Input: part model. Units: mm. Frame: model coordinates. Face numbers are marked on the shaded views. A direction names the side the tool comes from. Coordinates: 2 decimals unless noted, no trailing zeros. Order: outer loops, then holes, each group sorted by start corner. A loop starts at its lowest first (then second) coordinate and runs counter-clockwise, first axis right, second up. Notation, with made-up numbers: M 76,5.25 L 85,5.25 A5 cw 85,11.25 Z; hole C 44,55 d1. An arc over 180 degrees is marked long. Answer in a Markdown table with one row per item.
Autodesk Inventor part; units mm, degrees
ref_plane "YZ Plane" through (0, 0, 0) normal (1, 0, 0) x (0, 1, 0)
ref_plane "XZ Plane" through (0, 0, 0) normal (0, 1, 0) x (-1, 0, 0)
ref_plane "XY Plane" through (0, 0, 0) normal (0, 0, 1) x (1, 0, 0)
sketch "스케치1" plane through (0, 0, 0) normal (0, 0, 1) x (1, 0, 0)
  line L0 (-46, -31.5) -> (46, -31.5)
  line L1 (46, -31.5) -> (46, 31.5)
  line L2 (46, 31.5) -> (-46, 31.5)
  line L3 (-46, 31.5) -> (-46, -31.5)
  line L4 (-46, -31.5) -> (46, 31.5) construction
  line L5 (46, -31.5) -> (-46, 31.5) construction
  line L6 (-42.5, 28) -> (42.5, 28) construction
  line L7 (42.5, 28) -> (42.5, -28) construction
  line L8 (42.5, -28) -> (-42.5, -28) construction
  line L9 (-42.5, -28) -> (-42.5, 28) construction
  line L10 (-42.5, 28) -> (42.5, -28) construction
  line L11 (42.5, 28) -> (-42.5, -28) construction
  circle A0 centre (-39, -24.5) radius 1
  circle A1 centre (19, -24.5) radius 1
  line L12 (0, 0) -> (14.8173, 0)
  circle A2 centre (-39, 24.5) radius 1
  circle A3 centre (19, 24.5) radius 1
  line L13 (-46, 31.5) -> (-41, 31.5)
  line L14 (-41, 31.5) -> (-41, 34)
  line L15 (-41, 34) -> (-46, 34) construction
  line L16 (-46, 34) -> (-46, 31.5)
  circle A4 centre (-43.5, 34) radius 2.5
  circle A5 centre (-43.5, 34) radius 1.25
  line L17 (0, 0) -> (0, 10.4922)
  line L18 (46, 31.5) -> (41, 31.5)
  line L19 (41, 31.5) -> (41, 34)
  line L20 (41, 34) -> (46, 34) construction
  line L21 (46, 34) -> (46, 31.5)
  circle A6 centre (43.5, 34) radius 2.5
  circle A7 centre (43.5, 34) radius 1.25
  line L22 (46, -31.5) -> (-46, -31.5)
  line L23 (-46, -31.5) -> (-41, -31.5)
  line L24 (-41, -31.5) -> (-41, -34)
  line L25 (-41, -34) -> (-46, -34) construction
  line L26 (-46, -34) -> (-46, -31.5)
  circle A8 centre (-43.5, -34) radius 2.5
  circle A9 centre (-43.5, -34) radius 1.25
  line L27 (41, -31.5) -> (41, -34)
  circle A10 centre (43.5, -34) radius 1.25
  line L28 (41, -34) -> (46, -34) construction
  line L29 (46, -34) -> (46, -31.5)
  circle A11 centre (43.5, -34) radius 2.5
  line L30 (46, -31.5) -> (41, -31.5)
  dimension "d0" = 92
  dimension "d1" = 63
  dimension "d2" = 85
  dimension "d3" = 56
  dimension "d4" = 3.5
  dimension "d5" = 3.5
  dimension "d6" = 2
  dimension "d7" = 2
  dimension "d8" = 58
  dimension "d9" = 3.5
  dimension "d10" = 5
  dimension "d11" = 2.5
  dimension "d12" = 2.5
extrude "돌출1" add sketch "스케치1" along normal blind 4
sketch "스케치3" plane through (0, 0, 0) normal (0, 0, -1) x (-1, 0, 0)
  circle A0 centre (-19, 24.5) radius 1
  circle A1 centre (-19, 24.5) radius 3
  circle A2 centre (39, 24.5) radius 1
  circle A3 centre (39, 24.5) radius 3
  circle A4 centre (-19, -24.5) radius 1
  circle A5 centre (-19, -24.5) radius 3
  circle A6 centre (39, -24.5) radius 1
  circle A7 centre (39, -24.5) radius 3
  point P0 (0, 0)
  dimension "d24" = 6
  dimension "d25" = 6
  dimension "d26" = 6
  dimension "d27" = 6
extrude "돌출3" add sketch "스케치3" along normal blind 2.5
extrude "돌출4" add sketch "스케치1" against normal blind 2.5 contours L24 A8 L0 | L0 A11 L27 | A8 L26 L0 | A8 | L0 L29 A11 | A11 | L16 A4 L2 | L2 A6 L21 | A4 L14 L2 | A4 | L2 L19 A6 | A6
fillet "모깎기1" radius 2 4 edges at (43.5, 31.5, 0) (-43.5, 31.5, 0) (43.5, -31.5, 0) (-43.5, -31.5, 0)
fillet "모깎기2" radius 1 4 edges at (22, 24.5, 0) (22, -24.5, 0) (-36, 24.5, 0) (-36, -24.5, 0)
sketch "스케치4" plane through (0, 0, 4) normal (0, 0, 1) x (1, 0, 0)
  line L0 (-46, 34) -> (-46, -34)
  line L1 (46, -29.5) -> (46, 29.5)
  line L2 (46, -34) -> (46, 34)
  line L3 (46, -20) -> (24, -20)
  line L4 (24, -20) -> (24, 10)
  line L5 (24, 10) -> (46, 10)
  line L6 (46, 10) -> (46, -20)
  line L7 (46, -20) -> (41, -20)
  line L8 (41, -20) -> (41, -23)
  line L9 (41, -23) -> (46, -23)
  line L10 (46, -23) -> (46, -20)
  line L11 (46, 10) -> (41, 10)
  line L12 (41, 10) -> (41, 12)
  line L13 (41, 12) -> (46, 12)
  line L14 (46, 12) -> (46, 10)
  point P0 (46, 0)
  point P1 (46, -20)
  point P2 (46, 10)
  point P3 (46, 0)
  dimension "d40" = 30
  dimension "d42" = 10
  dimension "d43" = 3
  dimension "d44" = 5
  dimension "d45" = 22
  dimension "d46" = 5
  dimension "d47" = 2
extrude "돌출5" cut sketch "스케치4" against normal blind 10
properties part number "라즈베리파이 고정 커버"
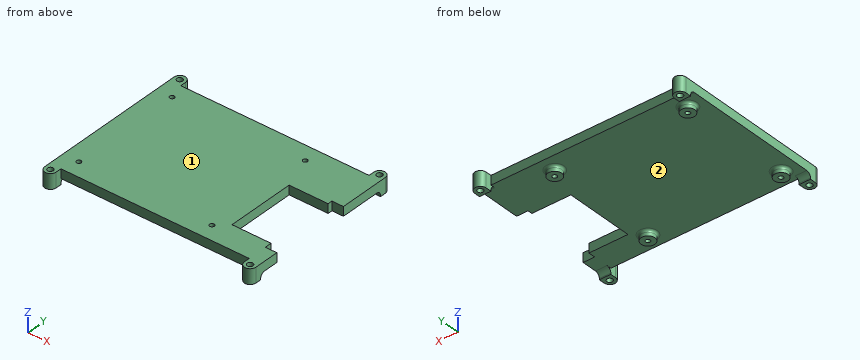
1) Reachability of the marked faces 1 and 2 from +Z, -Z, +X, -X, +Y, -Y: full face, straight path, thin tool, end or side. Return the list, or none.
Resolved:
| item | result |
|---|---|
| face 1 | +Z, +X, -X, +Y, -Y |
| face 2 | -Z |
2) Cut plane B-B, the plane y = 24.5. Output: boundary loops of the cut face in (x, z).
Resolved:
| item | result |
|---|---|
| outline | M -46,0 L -43,0 A1 cw -42,-1 L -42,-2.5 L -40,-2.5 L -40,4 L -46,4 Z; M -38,-2.5 L -36,-2.5 L -36,-1 A1 cw -35,0 L 15,0 A1 cw 16,-1 L 16,-2.5 L 18,-2.5 L 18,4 L -38,4 Z; M 20,-2.5 L 22,-2.5 L 22,-1 A1 cw 23,0 L 46,0 L 46,4 L 20,4 Z |
3) Cut plane A-A, the plane x = 43.5. Output: boundary loops of the cut face in (y, z).
Resolved:
| item | result |
|---|---|
| outline | M -36.5,-2.5 L -35.25,-2.5 L -35.25,4 L -36.5,4 Z; M -32.75,-2.5 L -31.5,-2.5 L -31.5,-2 A2 cw -29.5,0 L -23,0 L -23,4 L -32.75,4 Z; M 12,0 L 29.5,0 A2 cw 31.5,-2 L 31.5,-2.5 L 32.75,-2.5 L 32.75,4 L 12,4 Z; M 35.25,-2.5 L 36.5,-2.5 L 36.5,4 L 35.25,4 Z |
4) Contact query for flat-ended pins moving along their axis: pin 1 (2 mm diameter, centred on x = 29.5, z = 1, fed in from -Y); pin 2 (3 mm diameter, centred on x = -15, y = 6.5, fed in from -Z); pin 3 (3 mm diameter, centred on y = -3, z = 1.5, fed in from +X). Output: stop coordinate, or through.
Resolved:
| item | result |
|---|---|
| pin 1 | stops at y = -31.5 |
| pin 2 | stops at z = 0 |
| pin 3 | stops at x = 24 |
5) Cut plane C-C, the plane x = 19. Output: boundary loops of the cut face in (y, z), and give its area (3 significant figures).
Resolved:
| item | result |
|---|---|
| outline | M -31.5,0 L -28.5,0 A1 cw -27.5,-1 L -27.5,-2.5 L -25.5,-2.5 L -25.5,4 L -31.5,4 Z; M -23.5,-2.5 L -21.5,-2.5 L -21.5,-1 A1 cw -20.5,0 L 20.5,0 A1 cw 21.5,-1 L 21.5,-2.5 L 23.5,-2.5 L 23.5,4 L -23.5,4 Z; M 25.5,-2.5 L 27.5,-2.5 L 27.5,-1 A1 cw 28.5,0 L 31.5,0 L 31.5,4 L 25.5,4 Z |
| area | 257 mm2 |
6) Cut plane D-D, the plane z = 2.5. State how many separate pieces and enclosed holes the cut face has, and give its area (3 significant figures).
Resolved:
| item | result |
|---|---|
| separate pieces | 1 |
| enclosed holes | 8 |
| area | 5,170 mm2 |
7) Material intervals for probe 1 along Y at (x, z) = (-43.5, -1.75); probe 2 along Y at (x, z) = (19, -1.55); probe 3 along Y at (x, z) = (19, 1.05), sorted ascending.
Resolved:
| item | result |
|---|---|
| probe 1 | y = -36.5 to -35.25, -32.75 to -31.48, 31.48 to 32.75, 35.25 to 36.5 |
| probe 2 | y = -27.5 to -25.5, -23.5 to -21.5, 21.5 to 23.5, 25.5 to 27.5 |
| probe 3 | y = -31.5 to -25.5, -23.5 to 23.5, 25.5 to 31.5 |
